Answer from the drawing. Dimensions are ordinates in mm from the lowest x, y and z of the part. A direction names the side the tool comes from. Round coordinates to 2 decimals unless told otherwise and drop trailing zeros. Loops run counter-clockwise (first coordinate to the right, second up) from the corner with the lowest first, then second, coordinate; pieces in that order, holes last.
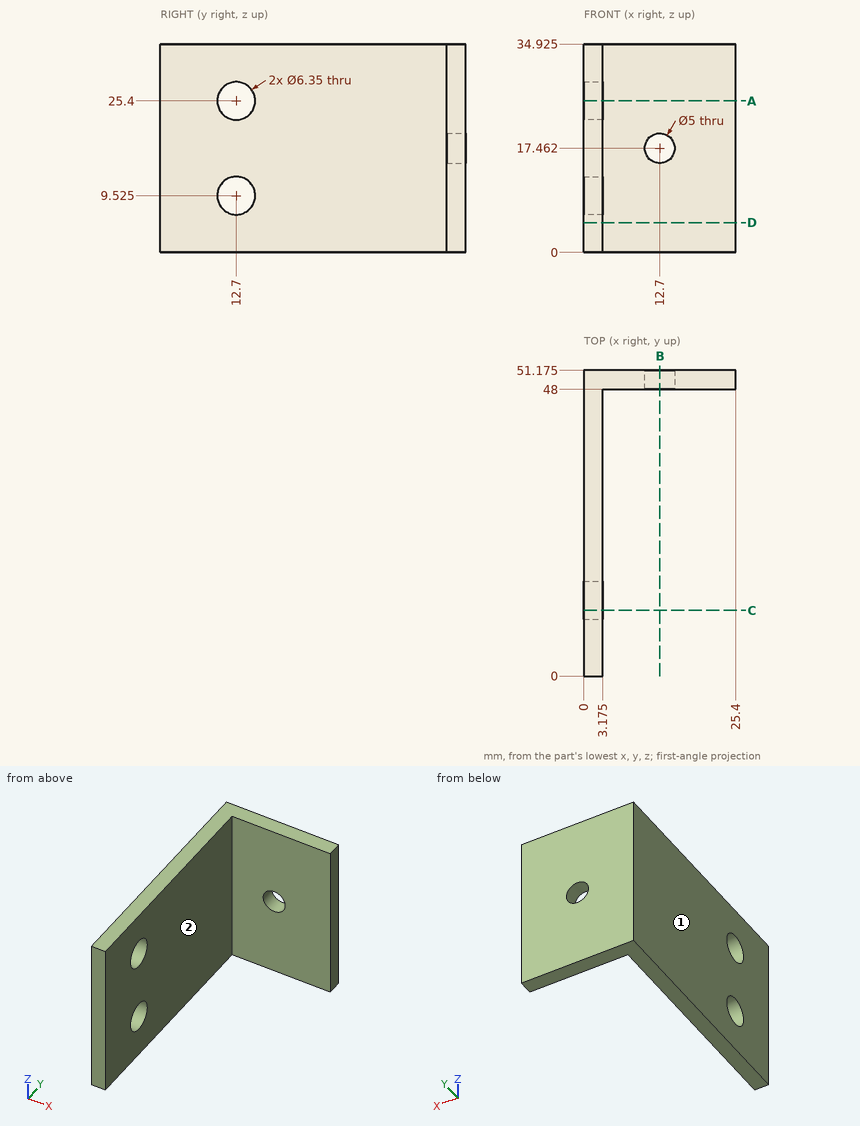
1. Consider probe 1 along Y at (x, z) = (1.95, 25.4) (1 decimal); probe 2 along Z at (x, y) = (12.7, 49.1) (1 decimal); probe 3 along X at (y, z) = (47, 5.5) (1 decimal). Determine where each line is inside the solid, lowest interval first.
Answer key:
probe 1: y = 0 to 9.5, 15.9 to 51.2
probe 2: z = 0 to 15, 20 to 34.9
probe 3: x = 0 to 3.2
2. Find section D-D (z = 5). Write down the section's boundary in (x, y) (1 decimal).
Answer key:
outline: (0, 0) - (3.2, 0) - (3.2, 48) - (25.4, 48) - (25.4, 51.2) - (0, 51.2) - close
3. Which of the six approach directions +Z, -Z, +X, -X, +Y, -Y give full straight-line access (tool end or side, diameter ignored) to the marked faces 1 and 2?
Answer key:
face 1: +Z, -Z, -X, +Y, -Y
face 2: +Z, -Z, +X, -Y
4. Find section A-A (z = 25.4). Write down the section's boundary in (x, y) (1 decimal), then the cut area to 3 significant figures.
Answer key:
outline: (0, 0) - (3.2, 0) - (3.2, 9.5) - (0, 9.5) - close; (0, 15.9) - (3.2, 15.9) - (3.2, 48) - (25.4, 48) - (25.4, 51.2) - (0, 51.2) - close
area: 213 mm2
5. Find section B-B (x = 12.7). Write down the section's boundary in (y, z) (1 decimal).
Answer key:
outline: (48, 0) - (51.2, 0) - (51.2, 15) - (48, 15) - close; (48, 20) - (51.2, 20) - (51.2, 34.9) - (48, 34.9) - close
6. Given pin 1 (6.5 mm diameter, centred on x = 18.5, z = 22, fed in from -Y); pin 2 (5.5 mm diameter, centred on y = 12.7, z = 9.525, fed in from +X); pin 3 (3 mm diameter, centred on y = 29.5, z = 8, fed in from +X) (1 decimal), each flat-ended and moving along its own axis, determine where each tip first touches the part or whether it passes through.
Answer key:
pin 1: stops at y = 48
pin 2: passes through
pin 3: stops at x = 3.2
7. Find section C-C (y = 11). Write down the section's boundary in (x, z) (1 decimal).
Answer key:
outline: (0, 0) - (3.2, 0) - (3.2, 6.8) - (0, 6.8) - close; (0, 12.2) - (3.2, 12.2) - (3.2, 22.7) - (0, 22.7) - close; (0, 28.1) - (3.2, 28.1) - (3.2, 34.9) - (0, 34.9) - close
